Geometry: final body of the model. Coordinates: model frame, mm. A direction names the side the tool comes from. Give positions to 0.01 mm unless a question says otherwise; leave off trailing zeros. Loops run counter-clockwise (first coordinate to the right, second up) from the corner with the lowest first, then second, coordinate; pieces in that order, holes last. Notation, with made-up numbers: (84, 68.25) -> (100, 68.25) arc R7 ccw to (100, 81.25) -> close; hole circle Ø6 at (-4, -14). An arc over 180 degrees is marked (long way). Answer in a Markdown table with one row per item. Add a question column.
1) Line query: line 1 (X direction, y = -6.25, z = -7.25); line 2 (X direction, y = -7.25, z = -4.75); line 3 (X direction, y = -8.75, z = 3). Output: solid intervals per line, ascending. Write a range as from..to.
2) Section query A-A (y = 0). Return the cut outline in (x, z), plus the area to 3 significant figures.
3) Draft query along X for faces 1 (the flat face through (5, -8.2, 0)), 2 (the cylindrical face through (52.99, 9.274, -2.059)), 3 (the flat face through (89.5, 0, 0)). Return one class per face: +X half, -X half, draft (parallel to the pull), parting line (faces both ways), or undercut.
4) First-contact query: P1, Ø3, axis at x = 32.5, y = -1, coming from the -Z side; P2, Ø10, axis at x = 19.5, z = 3.5, coming from the -Y side; P3, Ø1, axis at x = 37, z = -8, coming from the -Y side. Flat tips, straight axial feed; report the tip coordinate or a pass-through.
5) Access query for faces 4 (the conical face through (89, 0, -8)), 5 (the cylindrical face through (10.58, 7.81, -1.73)). Directions: +Z, -Z, +X, -X, +Y, -Y. A direction counts if a zero-diameter tool reaches every point of the face in a straight line with its end or side. Return the directions, or none.
6) Section query C-C (x = 46). Return the cut outline in (y, z), plus the area to 3 significant figures.
```python
from build123d import *


with BuildPart() as part:
    # Sketch1 → Revolve1 (revolve)
    with BuildSketch(Plane.XY, mode=Mode.PRIVATE) as revolve1_sk:
        with BuildLine():
            Line((0, 0), (0, 10))
            ThreePointArc((0, 10), (2.5, 12.5), (5, 10))
            Line((5, 10), (5, 8))
            Line((5, 8), (16, 8))
            ThreePointArc((16, 8), (16.439339828, 9.060660172), (17.5, 9.5))
            Line((17.5, 9.5), (87.5, 9.5))
            Line((87.5, 9.5), (89.5, 7.5))
            Line((89.5, 7.5), (89.5, 0))
            Line((89.5, 0), (0, 0))
        make_face()
    revolve(revolve1_sk.sketch.rotate(Axis((0, 0, 0), (1, 0, 0)), 90), axis=Axis((0, 0, 0), (1, 0, 0)))


solid = part.part
```
Evaluation:
| question | item | result |
|---|---|---|
| 1 | line 1 | 0..5 |
| 1 | line 2 | 0..5, 16.16..88.33 |
| 1 | line 3 | 0..5, 16.67..87.75 |
| 2 | outline | (0, -10) arc R2.5 ccw to (5, -10) -> (5, -8) -> (16, -8) arc R1.5 ccw to (17.5, -9.5) -> (87.5, -9.5) -> (89.5, -7.5) -> (89.5, 7.5) -> (87.5, 9.5) -> (17.5, 9.5) arc R1.5 ccw to (16, 8) -> (5, 8) -> (5, 10) arc R2.5 ccw to (0, 10) -> close |
| 2 | area | 1,690 mm² |
| 3 | face 1 | undercut |
| 3 | face 2 | draft |
| 3 | face 3 | +X half |
| 4 | P1 | z = -9.5 |
| 4 | P2 | y = -9.5 |
| 4 | P3 | y = -5.83 |
| 5 | face 4 | +X |
| 5 | face 5 | none |
| 6 | outline | circle Ø19 at (0, 0) |
| 6 | area | 284 mm² |
